Study the drawing (mm; zero at the part's minimum x, y, z) and answer. A direction names the side the tool comes from. Round coordinates to 2 decimals unless told otherwise and drop trailing zeros. Order: outer loops, then holes, each group sorted by start corner. A loop starts at its lowest first (then second) coordinate and runs counter-clockwise, first axis right, second up. Notation, with made-up numbers: M -1,30 L 56,30 A21 ccw 56,56 Z; hole C 39,39 d11. An arc over 180 degrees is marked long. Put each result on its own line as item: value. Start each with the question number.
1. The part is cut by section D-D (y = 8). Give the vertices of the cut face in (x, z), then the cut area to 3 significant figures.
2. Each of these flat-tipped pins is pushed along its axis until it touches: pin 1 Ø4 at (x, y) = (8.5, 3.5) entering from -Z; pin 2 Ø3 at (x, z) = (6.5, 12.5) entering from -Y; pin 3 Ø2 at (y, z) = (5, 13.5) entering from +X; pin 4 Ø3 at (x, y) = (4.5, 5) entering from +Z. Where does it stop, or does it pass through?
3. The part is cut by section A-A (z = 5). Give the vertices of the cut face in (x, y).
4. The part is cut by section B-B (x = 8.5). Give the vertices of the cut face in (y, z).
5. Consider line 1 (Y direction, x = 1, z = 15.75); line 2 (Y direction, x = 8, z = 5); line 3 (Z direction, x = 4, y = 5). Determine where each line is inside the solid, lowest interval first.
6. Which of the six approach directions +Z, -Z, +X, -X, +Y, -Y give full straight-line access (tool end or side, diameter ignored) to the marked faces 5 and 6?
7. The part is cut by section C-C (z = 13.5). Give the vertices of the cut face in (x, y).
8. The mould has two halves that part along Y. Classify the marked faces 1, 2, 3 and 4: +Y half, -Y half, draft (parallel to the pull), parting line (faces both ways), or undercut.
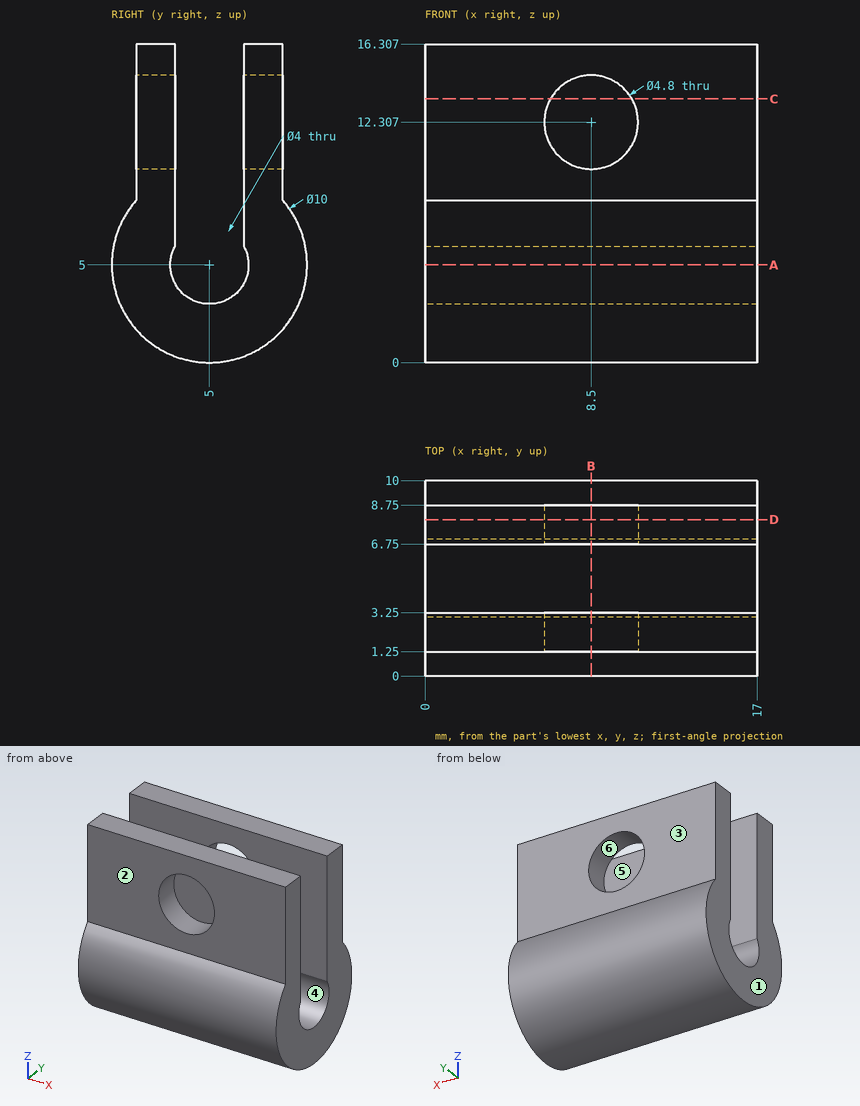
Resolved:
1. outline: M 0,1 L 17,1 L 17,16.31 L 0,16.31 Z; hole C 8.5,12.31 d4.8
1. area: 242 mm2
2. pin 1: z = 0
2. pin 2: y = 1.25
2. pin 3: through
2. pin 4: z = 3.68
3. outline: M 0,0 L 17,0 L 17,3 L 0,3 Z; M 0,7 L 17,7 L 17,10 L 0,10 Z
4. outline: M 1.25,8.31 A5 ccw long 8.75,8.31 L 8.75,9.91 L 6.75,9.91 L 6.75,5.97 A2 cw long 3.25,5.97 L 3.25,9.91 L 1.25,9.91 Z; M 1.25,14.71 L 3.25,14.71 L 3.25,16.31 L 1.25,16.31 Z; M 6.75,14.71 L 8.75,14.71 L 8.75,16.31 L 6.75,16.31 Z
5. line 1: 1.25 to 3.25, 6.75 to 8.75
5. line 2: 0 to 3, 7 to 10
5. line 3: 0 to 3
6. face 5: +Z, +X, -X
6. face 6: +Y, -Y
7. outline: M 0,1.25 L 6.42,1.25 L 6.42,3.25 L 0,3.25 Z; M 0,6.75 L 6.42,6.75 L 6.42,8.75 L 0,8.75 Z; M 10.58,1.25 L 17,1.25 L 17,3.25 L 10.58,3.25 Z; M 10.58,6.75 L 17,6.75 L 17,8.75 L 10.58,8.75 Z
8. face 1: draft
8. face 2: -Y half
8. face 3: +Y half
8. face 4: undercut
